Read the model definition and answer for the solid it produces. Units are mm, in the model's axes. A direction names the side the tool comes from. Round coordinates to 2 decimals unless told otherwise and drop trailing zeros. Order: outer loops, then holes, each group sorted by start corner. A loop starts at its lowest first (then second) coordinate and runs counter-clockwise, first axis right, second up. Notation, with made-up numbers: (-21.5, 12.5) - (13.5, 12.5) arc R22 ccw to (13.5, 49.5) - close; hole circle Ø8 at (-6, 72.25). An arc over 180 degrees is marked (long way). Answer as a JSON object with one key per item and string values. Group by question number.
Q1. A cutting plane is placed at A-A on z = -15. Determine the outline of the cut face in (x, y).
Q2. Given pin 1 Ø5 at (x, z) = (35.5, -15) entering from +Y; pin 2 Ø3 at (x, z) = (34.26, -15) entering from -Y; pin 3 Ø0.6 at (x, y) = (5.5, 0.5) entering from +Z; pin 4 Ø5 at (x, z) = (33, -28.5) entering from -Y, each flat-ended and moving along its own axis, determine where each tip first touches the part or whether it passes through.
Q3. A cutting plane is placed at D-D on z = -29. Determine the outline of the cut face in (x, y), and give its area (3 significant figures).
Q4. A cutting plane is placed at C-C on x = 18.5. Determine the outline of the cut face in (y, z), and give its area (3 significant figures).
Q5. Consider line 1 (X direction, y = 0.95, z = -15); line 2 (Y direction, x = 32, z = -10.5); line 3 (Z direction, x = 9, y = 0.9). Determine where each line is inside the solid, lowest interval first.
Q6. A tool of negligible diameter and unlimited length cuts with its end or side. For faces 1 (the flat face through (31.6, 1.5, -15.1)), 2 (the flat face through (15.5, 1, -35)), 3 (the flat face through (8, 1, 0)), from which of +Z, -Z, +X, -X, +Y, -Y can it reach the whole face along a straight path? Write none if from no direction.
Q7. The mould has two halves that part along X. Classify faces 4 (the flat face through (28, 4.77, -15)), 5 (the flat face through (15.5, 1, 5)), 6 (the cylindrical face through (28.857, 3.158, -16.084)): pulls with the +X half, pulls with the -X half, needs draft (parallel to the pull), parting line crosses it, or undercut.
Q8. A cutting plane is placed at B-B on y = 2.15. Determine the outline of the cut face in (x, z), and give its area (3 significant figures).
```python
from build123d import *

# Parameters (mm, degrees)
SALIENTE_EXTRUIR1_DEPTH = 4.77
CORTAR_EXTRUIR1_START   = -40
CROQUIS2_W              = 24.7
CROQUIS2_H              = 3.57
CORTAR_EXTRUIR1_DEPTH   = 50
CORTAR_EXTRUIR2_START   = -50
CORTAR_EXTRUIR2_DEPTH   = 50
CORTAR_EXTRUIR3_START   = -4.77
CROQUIS4_R              = 2.474873734
CORTAR_EXTRUIR3_DEPTH   = 4.77
CROQUIS5_R              = 5
CORTAR_EXTRUIR4_DEPTH   = 3.27


with BuildPart() as part:
    # Croquis1 → Saliente-Extruir1 (new body)
    with BuildSketch(Plane(origin=(0, 0, 0), x_dir=(1, 0, 0), z_dir=(0, 1, 0))):
        Polygon((0, 0), (15.5, 0), (15.5, -10), (45, -10), (45, 40), (15.5, 40), (15.5, 30), (0, 30), align=None)
    extrude(amount=SALIENTE_EXTRUIR1_DEPTH)

    # Croquis2 → Cortar-Extruir1 (cut)
    with BuildSketch(Plane.XY.offset(CORTAR_EXTRUIR1_START)):
        with Locations((12.35, 2.985)):
            Rectangle(CROQUIS2_W, CROQUIS2_H)
    extrude(amount=CORTAR_EXTRUIR1_DEPTH, mode=Mode.SUBTRACT)

    # Croquis3 → Cortar-Extruir2 (cut)
    with BuildSketch(Plane.XY.offset(10).offset(CORTAR_EXTRUIR2_START)):
        Polygon((45, 0), (36.738117648, 4.77), (45, 4.77), align=None)
    extrude(amount=CORTAR_EXTRUIR2_DEPTH, mode=Mode.SUBTRACT)

    # Croquis4 → Cortar-Extruir3 (cut)
    with BuildSketch(Plane(origin=(0, 4.77, 0), x_dir=(1, 0, 0), z_dir=(0, 1, 0)).offset(CORTAR_EXTRUIR3_START)):
        with Locations(Location((34.263243914, 15, 0), (0, 0, 270))):
            Circle(CROQUIS4_R)
    extrude(amount=CORTAR_EXTRUIR3_DEPTH, mode=Mode.SUBTRACT)

    # Croquis5 → Cortar-Extruir4 (cut)
    with BuildSketch(Plane(origin=(0, 4.77, 0), x_dir=(1, 0, 0), z_dir=(0, 1, 0))):
        with Locations(Location((33.738117648, 15, 0), (0, 0, 270))):
            Circle(CROQUIS5_R)
    extrude(amount=-CORTAR_EXTRUIR4_DEPTH, mode=Mode.SUBTRACT)


solid = part.part
```
Result set:
{
 "1": {"outline": "(0, 0) - (31.79, 0) - (31.79, 1.5) - (28.74, 1.5) - (28.74, 4.77) - (24.7, 4.77) - (24.7, 1.2) - (0, 1.2) - close; (36.74, 0) - (45, 0) - (38.74, 3.62) - (38.74, 1.5) - (36.74, 1.5) - close"},
 "2": {"pin 1": "stops at y = 1.5", "pin 2": "passes through", "pin 3": "stops at z = 0", "pin 4": "stops at y = 0"},
 "3": {"outline": "(0, 0) - (45, 0) - (36.74, 4.77) - (24.7, 4.77) - (24.7, 1.2) - (0, 1.2) - close", "area": "107 mm²"},
 "4": {"outline": "(0, -40) - (1.2, -40) - (1.2, 10) - (0, 10) - close", "area": "60.0 mm²"},
 "5": {"line 1": "x = 0 to 31.79, 36.74 to 43.35", "line 2": "y = 0 to 1.5", "line 3": "z = -30 to 0"},
 "6": {"face 1": "+Y", "face 2": "-Z, -X, +Y, -Y", "face 3": "+Z, -X, +Y, -Y"},
 "7": {"face 4": "needs draft", "face 5": "pulls with the -X half", "face 6": "undercut"},
 "8": {"outline": "(24.7, -40) - (41.28, -40) - (41.28, 10) - (24.7, 10) - close; hole circle Ø10 at (33.74, -15)", "area": "750 mm²"}
}
